```python
from build123d import *

# Parameters (mm, degrees)
SKETCH1_R           = 30
SKETCH1_R_2         = 7
BOSS_EXTRUDE1_DEPTH = 10
FILLET1_R           = 20
FILLET2_R           = 10
CUT_EXTRUDE1_DEPTH  = 161.838428244


with BuildPart() as part:
    # Sketch1 → Boss-Extrude1 (new, symmetric)
    with BuildSketch(Plane.XY):
        with BuildLine():
            Line((27.935473676, 25.760615491), (128.063755469, 9.084385863))
            ThreePointArc((128.063755469, 9.084385863), (155, 0), (128.063755469, -9.084385863))
            Line((128.063755469, -9.084385863), (27.935473676, -25.760615491))
            ThreePointArc((27.935473676, -25.760615491), (-38, 0), (27.935473676, 25.760615491))
        make_face()
        Circle(SKETCH1_R, mode=Mode.SUBTRACT)
        with Locations((140, 0)):
            Circle(SKETCH1_R_2, mode=Mode.SUBTRACT)
    extrude(amount=BOSS_EXTRUDE1_DEPTH, both=True)

    # Fillet1
    fillet1_edges = [part.edges().sort_by_distance(p)[0] for p in [
        (27.935473676, 25.760615491, 0),
        (27.935473676, -25.760615491, 0),
    ]]
    fillet(fillet1_edges, radius=FILLET1_R)

    # Fillet2
    fillet2_edges = [part.edges().sort_by_distance(p)[0] for p in [
        (128.063755469, 9.084385863, 0),
        (128.063755469, -9.084385863, 0),
    ]]
    fillet(fillet2_edges, radius=FILLET2_R)

    # Sketch3 → Cut-Extrude1 (cut, through all)
    with BuildSketch(Plane.XY.offset(10)):
        with BuildLine():
            Line((43.682358904, 16.548459765), (110.46878882, 5.425270378))
            ThreePointArc((110.46878882, 5.425270378), (115.065217391, 0), (110.46878882, -5.425270378))
            Line((110.46878882, -5.425270378), (43.682358904, -16.548459765))
            ThreePointArc((43.682358904, -16.548459765), (38.289832111, -14.701838037), (36.874374898, -9.180439854))
            ThreePointArc((36.874374898, -9.180439854), (38, 0), (36.874374898, 9.180439854))
            ThreePointArc((36.874374898, 9.180439854), (38.289832111, 14.701838037), (43.682358904, 16.548459765))
        make_face()
    extrude(amount=-CUT_EXTRUDE1_DEPTH, mode=Mode.SUBTRACT)


solid = part.part
```
Geometry check sheet. Reference: the model listing, model coordinates, mm. A direction names the side the tool comes from. Coordinates: 2 decimals unless noted, no trailing zeros. Order: outer loops, then holes, each group sorted by start corner. A loop starts at its lowest first (then second) coordinate and runs counter-clockwise, first axis right, second up. Notation, with made-up numbers: M 17.5,20.25 L 44.5,20.25 A27 ccw 44.5,56.25 Z; hole C -24.5,-8.75 d6. An arc over 180 degrees is marked long. Answer as a JSON object with one key per item and string values.
Q1. Depth check by flat-ended pin: pin 1 Ø10 at (x, z) = (110, -3.5) entering from -Y; pin 2 Ø2 at (y, z) = (6.5, -2.5) entering from +X; pin 3 Ø8 at (y, z) = (11.5, 2) entering from -X; pin 4 Ø11 at (x, y) = (140, 0) entering from -Z. Enter the tip coordinate at first touch or a pass-through.
Results are:
{"pin 1": "stops at y = -12.93", "pin 2": "stops at x = 153.96", "pin 3": "stops at x = -37.25", "pin 4": "passes through"}
Q2. Tool access check on faces 1 (the cylindrical face through (28.9, -26.3, 0.1)), 2 (the cylindrical face through (38, 0, 0)), 3 (the flat face through (77.872, 17.444, 0.14)), 4 (the flat face through (37.5, 3, 10)), 5 (the flat face through (79.12, -17.236, 0.14)). Record the directions out of +Z, -Z, +X, -X, +Y, -Y that give a thin tool (end or side, any length) a straight path to the whole face; none if there is none.
Results are:
{"face 1": "+Z, -Z, +X, -Y", "face 2": "+Z, -Z", "face 3": "+Z, -Z, +Y", "face 4": "+Z, +X, -X, +Y, -Y", "face 5": "+Z, -Z, -Y"}
Q3. Scan lines: line 1 (Y direction, x = 0, z = 4.75); line 2 (Y direction, x = 140, z = -1.25); line 3 (X direction, y = 4, z = 5). Record each from-to range of solid material in increasing order.
Results are:
{"line 1": "y = -38 to -30, 30 to 38", "line 2": "y = -15 to -7, 7 to 15", "line 3": "x = -37.79 to -29.73, 29.73 to 37.79, 113.34 to 134.26, 145.74 to 154.46"}
Q4. Cross-section at B-B on y = 0. Record the cut outline in (x, z), and give its area (3 significant figures).
Results are:
{"outline": "M -38,-10 L -30,-10 L -30,10 L -38,10 Z; M 30,-10 L 38,-10 L 38,10 L 30,10 Z; M 115.07,-10 L 133,-10 L 133,10 L 115.07,10 Z; M 147,-10 L 155,-10 L 155,10 L 147,10 Z", "area": "839 mm²"}
Q5. Cross-section at A-A on x = 0. Record the cut outline in (y, z), and give its area (3 significant figures).
Results are:
{"outline": "M -38,-10 L -30,-10 L -30,10 L -38,10 Z; M 30,-10 L 38,-10 L 38,10 L 30,10 Z", "area": "320 mm²"}
Q6. Release check for a two-part mould opening along X. For faces 6 (the cylindrical face through (28.9, 26.3, 0.1)), 7 (the flat face through (37.5, 3, -10)), 8 (the flat face through (77, 11, 0)), 9 (the cylindrical face through (-29.97, 1.32, -0.14)) record: released by +X, released by -X, zero draft, split by the parting line, or undercut.
Results are:
{"face 6": "released by +X", "face 7": "zero draft", "face 8": "undercut", "face 9": "undercut"}
Q7. Cross-section at C-C on z = 2. Record the cut outline in (x, y), and give its area (3 significant figures).
Results are:
{"outline": "M 24.38,-29.15 A20 cw 33.92,-24.76 L 123.07,-9.92 A10 cw 130.83,-11.87 A15 ccw long 130.83,11.87 A10 cw 123.07,9.92 L 33.92,24.76 A20 cw 24.38,29.15 A38 ccw long Z; hole C 0,0 d60; hole M 36.87,-9.18 A6 ccw 43.68,-16.55 L 110.47,-5.43 A5.5 ccw 110.47,5.43 L 43.68,16.55 A6 ccw 36.87,9.18 A38 cw Z; hole C 140,0 d14", "area": "3,670 mm²"}
Q8. Cross-section at D-D on x = 86.5. Record the cut outline in (y, z).
Results are:
{"outline": "M -16.01,-10 L -9.42,-10 L -9.42,10 L -16.01,10 Z; M 9.42,-10 L 16.01,-10 L 16.01,10 L 9.42,10 Z"}
